Part model, mm, in its own coordinate system. A direction names the side the tool comes from. Coordinates: 2 decimals unless noted, no trailing zeros. Write each loop counter-clockwise with the first axis right and the second up, starting at its lowest first coordinate (ties: lowest second). Pieces come first, ordered by that corner, then holes. Notation, with made-up numbers: (-19, 56.5) -> (0, 56.5) arc R19 cw to (0, 61.5) -> close; hole circle Ø1 at (-26, 5). An arc over 180 degrees is marked (long way). One line per question, with ' | ' between items. Start each with the question number.
Item 1: Saw through at A-A (y = 42). List the corners of the cut face in (x, z) (3 decimals).
Item 2: Probe probe 1 along X at (y, z) = (31.5, 74.5) (3 decimals); probe 2 along Y at (x, z) = (7.5, 101.5) (3 decimals). List the from-to ranges inside material, lowest first. Write a range as [from, to].
Item 3: Two-plate mould, pull along Z, no slides. Class faces 3 (the flat face through (64, 53.975, 66)), 4 (the flat face through (0, 27, 64)), 5 (the flat face through (3.175, 27, 64)), 6 (the flat face through (64, 27, 129.54)): pulls with the +Z half, pulls with the -Z half, needs draft (parallel to the pull), parting line crosses it, or undercut.
Item 4: Saw through at B-B (x = 89). List the corners of the cut face in (y, z) (3 decimals), and give its area (3 significant figures).
Item 5: 3-axis set-ups, long thin cutter, end or side, ignore diameter. For faces 1 (the flat face through (126.365, 27, 64)), 2 (the flat face through (64, 27, 0)): which of +Z, -Z, +X, -X, +Y, -Y reach the whole face in a straight line?
Item 6: Pin check, flat tip, straight feed: pin 1 (1 mm diameter, centred on x = 25, z = 86, fed in from -Y) (3 decimals). Stop position of the tip, or through.
Item 7: Saw through at C-C (z = 100). List the corners of the cut face in (x, y) (3 decimals), and give its area (3 significant figures).
from build123d import *

# Parameters (mm, degrees)
F0_W     = 129.54
F0_H     = 129.54
F1_DEPTH = 57.15
F2_T     = -3.175
F3_R     = 1.524
F4_R     = 1.524
F5_R     = 1.524


with BuildPart() as f1:
    # F0 (on Front) → F1 (new body)
    with BuildSketch(Plane.XZ):
        with Locations((64.77, 64.77)):
            Rectangle(F0_W, F0_H)
    extrude(amount=-F1_DEPTH)

    # F2
    f2_openings = [f1.faces().sort_by_distance(p)[0] for p in [
        (64.77, 0, 64.77),
    ]]
    offset(amount=F2_T, openings=f2_openings)

    # F3
    f3_edges = [f1.edges().sort_by_distance(p)[0] for p in [
        (3.175, 26.9875, 126.365),
        (64.77, 53.975, 126.365),
        (3.175, 53.975, 64.77),
        (3.175, 26.9875, 3.175),
        (64.77, 53.975, 3.175),
        (126.365, 53.975, 64.77),
        (126.365, 26.9875, 126.365),
        (126.365, 26.9875, 3.175),
    ]]
    fillet(f3_edges, radius=F3_R)

    # F4
    f4_edges = [f1.edges().sort_by_distance(p)[0] for p in [
        (129.54, 28.575, 0),
        (64.77, 57.15, 0),
        (129.54, 57.15, 64.77),
        (129.54, 28.575, 129.54),
        (64.77, 57.15, 129.54),
        (0, 28.575, 129.54),
        (0, 57.15, 64.77),
        (0, 28.575, 0),
    ]]
    fillet(f4_edges, radius=F4_R)

    # F5
    f5_edges = [f1.edges().sort_by_distance(p)[0] for p in [
        (64.77, 0, 3.175),
    ]]
    fillet(f5_edges, radius=F5_R)


solid = f1.part
From the geometry:
1) outline: (0, 1.524) arc R1.524 ccw to (1.524, 0) -> (128.016, 0) arc R1.524 ccw to (129.54, 1.524) -> (129.54, 128.016) arc R1.524 ccw to (128.016, 129.54) -> (1.524, 129.54) arc R1.524 ccw to (0, 128.016) -> close; hole (3.175, 4.699) arc R1.524 ccw to (4.699, 3.175) -> (124.841, 3.175) arc R1.524 ccw to (126.365, 4.699) -> (126.365, 124.841) arc R1.524 ccw to (124.841, 126.365) -> (4.699, 126.365) arc R1.524 ccw to (3.175, 124.841) -> close
2) probe 1: [0, 3.175], [126.365, 129.54] | probe 2: [53.975, 57.15]
3) face 3: undercut | face 4: needs draft | face 5: undercut | face 6: pulls with the +Z half
4) outline: (0, 0) -> (55.626, 0) arc R1.524 ccw to (57.15, 1.524) -> (57.15, 128.016) arc R1.524 ccw to (55.626, 129.54) -> (0, 129.54) -> (0, 127.889) arc R1.524 ccw to (1.524, 126.365) -> (52.451, 126.365) arc R1.524 cw to (53.975, 124.841) -> (53.975, 4.699) arc R1.524 cw to (52.451, 3.175) -> (1.524, 3.175) arc R1.524 ccw to (0, 1.651) -> close | area: 753 mm2
5) face 1: -Y | face 2: -Z, +X, -X, +Y, -Y
6) pin 1: y = 53.975
7) outline: (0, 0) -> (1.651, 0) arc R1.524 ccw to (3.175, 1.524) -> (3.175, 52.451) arc R1.524 cw to (4.699, 53.975) -> (124.841, 53.975) arc R1.524 cw to (126.365, 52.451) -> (126.365, 1.524) arc R1.524 ccw to (127.889, 0) -> (129.54, 0) -> (129.54, 55.626) arc R1.524 ccw to (128.016, 57.15) -> (1.524, 57.15) arc R1.524 ccw to (0, 55.626) -> close | area: 753 mm2
